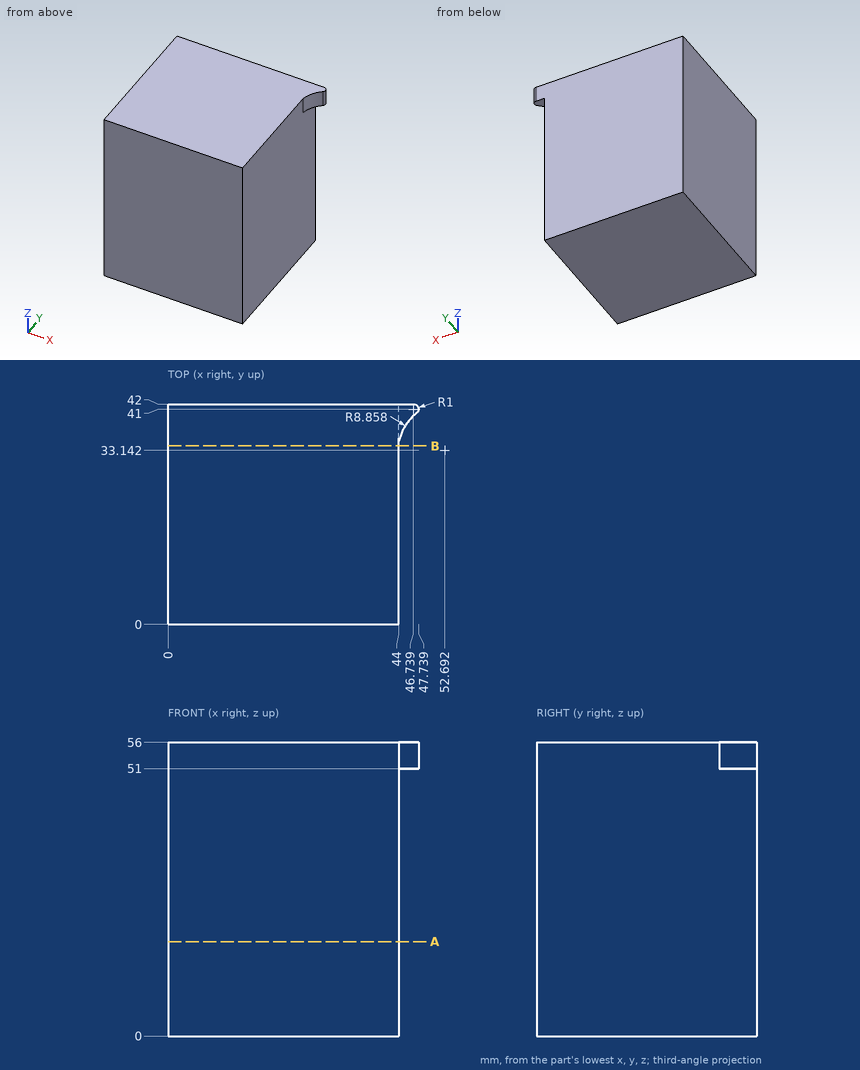
Job drawing, mm, ordinate dimensions from the low corner. One solid piece. Give positions to 0.01 mm unless a question says otherwise; leave off trailing zeros. Order: outer loops, then holes, each group sorted by start corner. A loop starts at its lowest first (then second) coordinate and runs counter-clockwise, first axis right, second up. Notation, with made-up numbers: M 49,54.25 L 59,54.25 A21 ccw 59,58.25 Z; hole C 87,57.5 d4. An arc over 180 degrees is marked long. Put each result on its own line as item: value. Start each with the question number.
(1) Drill centre line: L1, parallel to X at y = 21.5, z = 33.5. Where is it in solid material? Low to high. Write a range as [from, to].
(2) Band-saw the part on B-B on y = 34. Give the cut face in (x, z), then the cut area to 3 significant figures.
(3) Pin check, flat tips, straight feed: pin 1 Ø2 at (y, z) = (31, 37.5) entering from +X; pin 2 Ø1.1 at (x, y) = (46, 39) entering from -Z. Stop position of each tip, or through.
(4) Band-saw the part on A-A on z = 18. Give the cut face in (x, y), then the cut area to 3 significant figures.
Results below:
1. L1: x = [0, 44]
2. outline: M 0,0 L 44,0 L 44,56 L 0,56 Z
2. area: 2,460 mm2
3. pin 1: stops at x = 44
3. pin 2: stops at z = 51
4. outline: M 0,0 L 44,0 L 44,42 L 0,42 Z
4. area: 1,850 mm2
